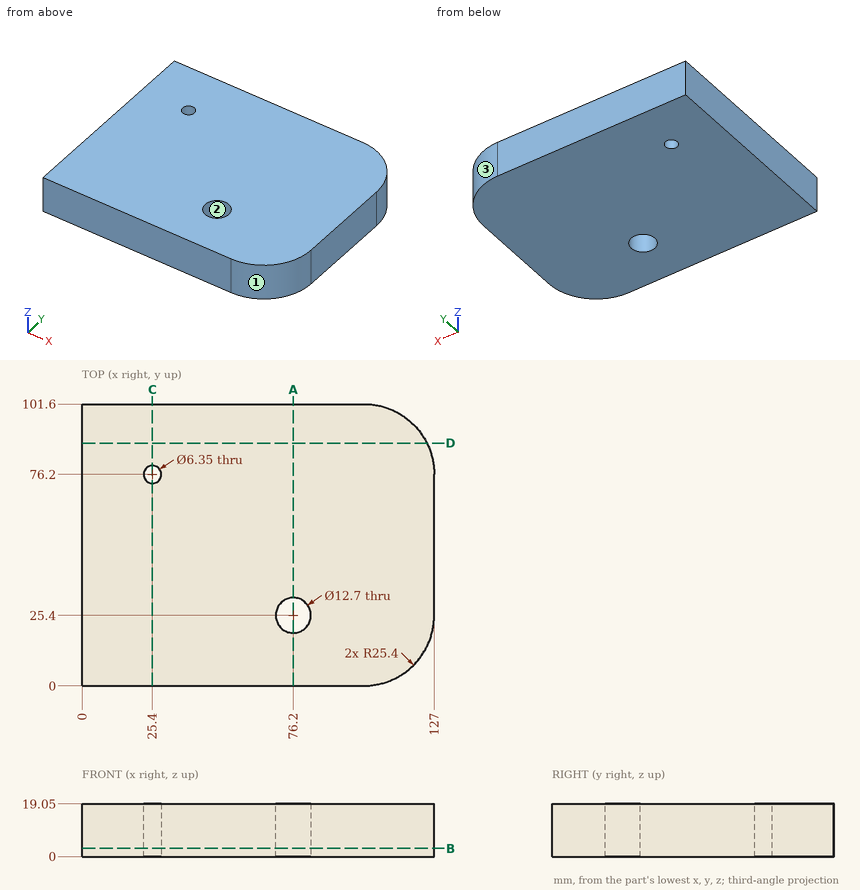
Input: dimensioned drawing with shaded views. Units: mm. Origin: part minimum x, y, z. Round coordinates to 2 decimals unless told otherwise and drop trailing zeros. Order: outer loops, then holes, each group sorted by start corner. A loop starts at its lowest first (then second) coordinate and runs counter-clockwise, first axis right, second up. Notation, with made-up numbers: (79.5, -29) -> (118.5, -29) arc R17 ccw to (118.5, -9) -> close; hole circle Ø5 at (28, 32.25). An arc over 180 degrees is marked (long way). One line per item, written item: value. Start each with the question number.
Q1. Draft query along Y for the marked faces 1, 2 and 3. Return one class per face: pulls with the +Y half, pulls with the -Y half, needs draft (parallel to the pull), parting line crosses it, or undercut.
Q2. Material intervals for probe 1 along X at (y, z) = (26, 7.25); probe 2 along Y at (x, z) = (76.2, 13.25); probe 3 along Y at (x, z) = (25.4, 10.25) (3 decimals), sorted ascending.
Q3. Section query A-A (x = 76.2). Return the cut outline in (y, z), plus the area to 3 significant figures.
Q4. Section query B-B (z = 3). Return the cut outline in (x, y) (3 decimals), plus the area to 3 significant figures.
Q5. Section query D-D (y = 87.5). Return the cut outline in (x, z).
Q6. Pin query (flat end, axial travel): pin 1 (5.5 mm diameter, centred on x = 25.4, y = 76.2, fed in from +Z); pin 2 (2 mm diameter, centred on y = 89.5, z = 5.5, fed in from +X). Return the tip coordinate at first contact, or that it passes through.
Q7. Section query C-C (x = 25.4). Return the cut outline in (y, z) (3 decimals), plus the area to 3 significant figures.
Findings below:
1. face 1: pulls with the -Y half
1. face 2: undercut
1. face 3: pulls with the +Y half
2. probe 1: 0 to 69.88, 82.52 to 127
2. probe 2: 0 to 19.05, 31.75 to 101.6
2. probe 3: 0 to 73.025, 79.375 to 101.6
3. outline: (0, 0) -> (19.05, 0) -> (19.05, 19.05) -> (0, 19.05) -> close; (31.75, 0) -> (101.6, 0) -> (101.6, 19.05) -> (31.75, 19.05) -> close
3. area: 1,690 mm²
4. outline: (0, 0) -> (101.6, 0) arc R25.4 ccw to (127, 25.4) -> (127, 76.2) arc R25.4 ccw to (101.6, 101.6) -> (0, 101.6) -> close; hole circle Ø6.35 at (25.4, 76.2); hole circle Ø12.7 at (76.2, 25.4)
4. area: 12,500 mm²
5. outline: (0, 0) -> (124.35, 0) -> (124.35, 19.05) -> (0, 19.05) -> close
6. pin 1: through
6. pin 2: x = 123.82
7. outline: (0, 0) -> (73.025, 0) -> (73.025, 19.05) -> (0, 19.05) -> close; (79.375, 0) -> (101.6, 0) -> (101.6, 19.05) -> (79.375, 19.05) -> close
7. area: 1,810 mm²
